Model file for the job. Use its own axes, mm. Face numbers are marked on the shaded views. A direction names the side the tool comes from. Round coordinates to 2 decimals unless told otherwise and drop trailing zeros. Loops run counter-clockwise (first coordinate to the right, second up) from the corner with the lowest first, then second, coordinate; pieces in that order, holes last.
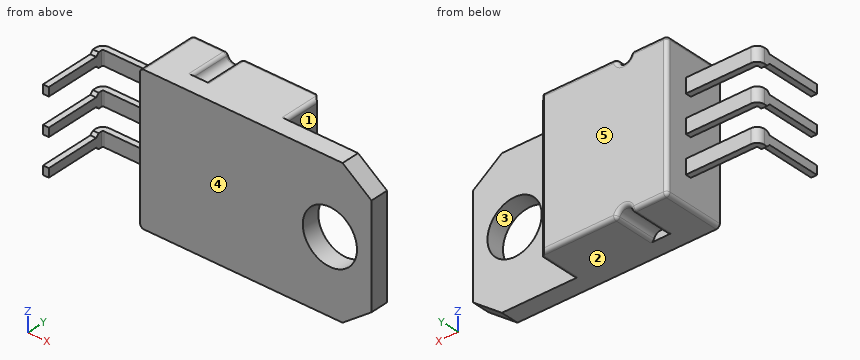
from build123d import *

# Parameters (mm, degrees)
SKETCH_1_R               = 1.875
EXTRUDE_1_DEPTH          = 1.25
EXTRUDE_2_DEPTH          = 3
FILLET_1_R               = 0.25
CHAMFER_1_SIZE           = 0.5
SKETCH_3_W               = 0.999690432
SKETCH_3_H               = 0.4
CUT_EXTRUDE_1_REACH      = 25.645
PATTERN_LINEAR_1_COUNT   = 2
PATTERN_LINEAR_1_PITCH   = 2.54
MIRROR_1_COPY_1_SKETCH_W = 0.999690432
MIRROR_1_COPY_1_SKETCH_H = 0.4
MIRROR_1_COPY_2_REACH    = 25.645


with BuildPart() as part:
    # Sketch 1 → Extrude 1 (new body)
    with BuildSketch(Plane(origin=(0, 0, 0), x_dir=(1, 0, 0), z_dir=(0, 1, 0))):
        Polygon((0, 0), (14, 0), (16, 1.5), (16, 8.5), (14, 10), (0, 10), align=None)
        with Locations(Location((13.125, 5, 0), (0, 0, 270))):
            Circle(SKETCH_1_R, mode=Mode.SUBTRACT)
    extrude(amount=EXTRUDE_1_DEPTH)

    # Sketch 2 → Extrude 2 (add)
    with BuildSketch(Plane(origin=(0, 1.25, 0), x_dir=(1, 0, 0), z_dir=(0, 1, 0))):
        with BuildLine():
            Line((0, 10), (2.5, 10))
            ThreePointArc((2.5, 10), (3, 9.5), (3.5, 10))
            Line((3.5, 10), (9, 10))
            Line((9, 10), (9, 0))
            Line((9, 0), (3.5, 0))
            ThreePointArc((3.5, 0), (3, 0.5), (2.5, 0))
            Line((2.5, 0), (0, 0))
            Line((0, 0), (0, 10))
        make_face()
    extrude(amount=EXTRUDE_2_DEPTH)

    # Fillet 1
    fillet_1_edges = [part.edges().sort_by_distance(p)[0] for p in [
        (0, 2.125, -10),
        (2.5, 2.75, -10),
        (3.5, 2.75, -10),
        (6.25, 4.25, -10),
        (3, 4.25, -9.5),
        (1.25, 4.25, -10),
        (0, 4.25, -5),
        (0, 2.125, 0),
        (3.5, 2.75, 0),
        (2.5, 2.75, 0),
        (1.25, 4.25, 0),
        (3, 4.25, -0.5),
        (6.25, 4.25, 0),
        (9, 2.75, -10),
        (9, 2.75, 0),
    ]]
    fillet(fillet_1_edges, radius=FILLET_1_R)

    # Chamfer 1
    # the kernel refuses this chamfer: 0.5 mm, written as the material it takes off along each edge
    with BuildSketch(Plane(origin=(9, 4.25, -11.035841494), x_dir=(-0.9996219169112968, 0.027495876610585647, 0), z_dir=(0, 0, 1))) as chamfer_1_piece_1:
        Polygon((CHAMFER_1_SIZE * 0.999621916911, CHAMFER_1_SIZE * 0.0274958766106), (-CHAMFER_1_SIZE * 0.0274958766106, CHAMFER_1_SIZE * 0.999621916911), (0, 0), align=None)
    extrude(amount=12.071682988, mode=Mode.SUBTRACT)

    # Sweep 1: sweep along a path in Sketch 4
    with BuildLine(Plane(origin=(0, 0, -5), x_dir=(-1, 0, 0), z_dir=(0, 0, -1))) as sweep_1_path:
        Line((0, 2.74), (4.5, 2.74))
        ThreePointArc((4.5, 2.74), (4.853553391, 2.593553391), (5, 2.24))
        Line((5, 2.24), (5, -2))
    # Sketch 3 → Sweep 1 (sweep)
    with BuildSketch(Plane.ZY):
        with Locations((-5, 2.54)):
            Rectangle(SKETCH_3_W, SKETCH_3_H)
    sweep_1 = sweep(path=sweep_1_path.line)

    # Sketch 5 → Cut-Extrude 1 (cut, up to next)
    with BuildSketch(Plane.ZY.offset(5), mode=Mode.PRIVATE) as cut_extrude_1_sk1:
        Polygon((-4.7, 1.814659855), (-4.7, -2), (-4.500154784, -2), (-4.500154784, 2.014505072), align=None)
    cut_extrude_1_tool1 = extrude(cut_extrude_1_sk1.sketch, amount=-CUT_EXTRUDE_1_REACH, mode=Mode.PRIVATE) & part.part
    # Sketch 5 → Cut-Extrude 1 (cut, up to next)
    with BuildSketch(Plane.ZY.offset(5), mode=Mode.PRIVATE) as cut_extrude_1_sk2:
        Polygon((-5.3, 1.814659855), (-5.3, -2), (-5.499845216, -2), (-5.499845216, 2.014505072), align=None)
    cut_extrude_1_tool2 = extrude(cut_extrude_1_sk2.sketch, amount=-CUT_EXTRUDE_1_REACH, mode=Mode.PRIVATE) & part.part
    cut_extrude_1_1 = cut_extrude_1_tool1.solids().sort_by_distance((-5, -0.042284, -4.599227))[0]
    add(cut_extrude_1_1, mode=Mode.SUBTRACT)
    cut_extrude_1_2 = cut_extrude_1_tool2.solids().sort_by_distance((-5, -0.042284, -5.400773))[0]
    add(cut_extrude_1_2, mode=Mode.SUBTRACT)
    cut_extrude_1 = cut_extrude_1_1 + cut_extrude_1_2  # Cut-Extrude 1 as one shape, for the pattern or mirror that repeats it

    # Pattern Linear 1: Sweep 1, Cut-Extrude 1 ×2
    with Locations(*[(0, 0, i * PATTERN_LINEAR_1_PITCH) for i in range(1, PATTERN_LINEAR_1_COUNT)]):
        add(sweep_1)
        add(cut_extrude_1, mode=Mode.SUBTRACT)

    # Mirror 1: Sweep 1, Cut-Extrude 1 across plane
    add(sweep_1.mirror(Plane(origin=(0, 0, -5), x_dir=(1, 0, 0), z_dir=(0, 0, -1))))
    add(cut_extrude_1.mirror(Plane(origin=(0, 0, -5), x_dir=(1, 0, 0), z_dir=(0, 0, -1))), mode=Mode.SUBTRACT)

    # Mirror 1 copy 1: sweep along a path in Mirror 1 copy 1 path
    with BuildLine(Plane(origin=(0, 0, -7.54), x_dir=(-1, 0, 0), z_dir=(0, 0, 1))) as mirror_1_copy_1_path:
        Line((0, -2.74), (4.5, -2.74))
        ThreePointArc((4.5, -2.74), (4.853553391, -2.593553391), (5, -2.24))
        Line((5, -2.24), (5, 2))
    # Mirror 1 copy 1 sketch → Mirror 1 copy 1 (sweep)
    with BuildSketch(Plane(origin=(0, 0, -12.54), x_dir=(0, 0, -1), z_dir=(-1, 0, 0))):
        with Locations((-5, -2.54)):
            Rectangle(MIRROR_1_COPY_1_SKETCH_W, MIRROR_1_COPY_1_SKETCH_H)
    sweep(path=mirror_1_copy_1_path.line)

    # Mirror 1 copy 2 sketch → Mirror 1 copy 2 (cut, up to next)
    with BuildSketch(Plane(origin=(-5, 0, -12.54), x_dir=(0, 0, -1), z_dir=(-1, 0, 0)), mode=Mode.PRIVATE) as mirror_1_copy_2_sk1:
        Polygon((-4.7, -1.814659855), (-4.7, 2), (-4.500154784, 2), (-4.500154784, -2.014505072), align=None)
    mirror_1_copy_2_tool1 = extrude(mirror_1_copy_2_sk1.sketch, amount=-MIRROR_1_COPY_2_REACH, mode=Mode.PRIVATE) & part.part
    # Mirror 1 copy 2 sketch → Mirror 1 copy 2 (cut, up to next)
    with BuildSketch(Plane(origin=(-5, 0, -12.54), x_dir=(0, 0, -1), z_dir=(-1, 0, 0)), mode=Mode.PRIVATE) as mirror_1_copy_2_sk2:
        Polygon((-5.3, -1.814659855), (-5.3, 2), (-5.499845216, 2), (-5.499845216, -2.014505072), align=None)
    mirror_1_copy_2_tool2 = extrude(mirror_1_copy_2_sk2.sketch, amount=-MIRROR_1_COPY_2_REACH, mode=Mode.PRIVATE) & part.part
    add(mirror_1_copy_2_tool1.solids().sort_by_distance((-5, -0.042284, -7.940773))[0], mode=Mode.SUBTRACT)
    add(mirror_1_copy_2_tool2.solids().sort_by_distance((-5, -0.042284, -7.139227))[0], mode=Mode.SUBTRACT)


solid = part.part
Q1. Slice it at D-D on z = -7.5. Give the cut face in (x, y).
Q2. Slice it at C-C on y = -1. Give the cut face in (x, z).
Q3. Flat gauge pins, fed straight in: P1, Ø1.1, axis at x = -2.5, z = -2.5, coming from the +Y side; P2, Ø2, axis at x = 10.5, z = -8, coming from the +Y side; P3, Ø3, axis at y = 3, z = -5.5, coming from the +X side. Where does each tip first touch, or does it go through?
Q4. Tool access for the marked faces 4 and 5: list every direction of +Z, -Z, +X, -X, +Y, -Y with a clear straight run to the whole face (end or side of a thin tool).
Q5. Slice it at A-A on y = 0.75. Give the cut face in (x, z) (3 decimals), plus the area to 3 significant figures.
Q6. Slice it at B-B on z = -5. Give the cut face in (x, y), plus the area to 3 significant figures.
Q7. Probe line 1 (Z direction, x = -0.25, y = 2.5); line 2 (X direction, y = 0.5, z = -5); line 3 (X direction, y = 2, z = -7.5). List the from-to ranges inside material, lowest first.
Q8. Pull direction Z, two halves, no side cores. Call the marked faces 1, 2 and 3: pulls with the +Z half, pulls with the -Z half, needs draft (parallel to the pull), parting line crosses it, or undercut.
Reply:
1. outline: (-5, -2) - (-4.6, -2) - (-4.6, 2.24) arc R0.1 cw to (-4.5, 2.34) - (0, 2.34) - (0, 0) - (16, 0) - (16, 1.25) - (9, 1.25) - (9, 3.75) - (8.5, 4.25) - (0.25, 4.25) arc R0.25 ccw to (0, 4) - (0, 2.74) - (-4.5, 2.74) arc R0.5 ccw to (-5, 2.24) - close
2. outline: (-5, -7.84) - (-4.6, -7.84) - (-4.6, -7.24) - (-5, -7.24) - close; (-5, -5.3) - (-4.6, -5.3) - (-4.6, -4.7) - (-5, -4.7) - close; (-5, -2.76) - (-4.6, -2.76) - (-4.6, -2.16) - (-5, -2.16) - close
3. P1: stops at y = 2.74
3. P2: stops at y = 1.25
3. P3: stops at x = 9
4. face 4: +Z, -Z, +X, -Y
4. face 5: +Z, -Z, +X, -X, +Y
5. outline: (-5, -7.84) - (-4.6, -7.84) - (-4.6, -7.24) - (-5, -7.24) - close; (-5, -5.3) - (-4.6, -5.3) - (-4.6, -4.7) - (-5, -4.7) - close; (-5, -2.76) - (-4.6, -2.76) - (-4.6, -2.16) - (-5, -2.16) - close; (0, -9.75) arc R0.25 ccw to (0.25, -10) - (14, -10) - (16, -8.5) - (16, -1.5) - (14, 0) - (0.25, 0) arc R0.25 ccw to (0, -0.25) - close; hole circle Ø3.75 at (13.125, -5)
5. area: 147 mm2
6. outline: (-5, -2) - (-4.6, -2) - (-4.6, 2.24) arc R0.1 cw to (-4.5, 2.34) - (0, 2.34) - (0, 0) - (11.25, 0) - (11.25, 1.25) - (9, 1.25) - (9, 3.75) - (8.5, 4.25) - (0.25, 4.25) arc R0.25 ccw to (0, 4) - (0, 2.74) - (-4.5, 2.74) arc R0.5 ccw to (-5, 2.24) - close; (15, 0) - (16, 0) - (16, 1.25) - (15, 1.25) - close
6. area: 45.9 mm2
7. line 1: z = -8.04 to -7.04, -5.5 to -4.5, -2.96 to -1.96
7. line 2: x = -5 to -4.6, 0 to 11.25, 15 to 16
7. line 3: x = -5 to -4.6, 0 to 9
8. face 1: needs draft
8. face 2: pulls with the -Z half
8. face 3: undercut
